from build123d import *

# Parameters (mm, degrees)
F1_DEPTH = 50.038
F3_W     = 44.874294
F3_H     = 28.605775
F4_DEPTH = 25.4


with BuildPart() as f1:
    # F0 (on Right) → F1 (new body)
    with BuildSketch(Plane.YZ):
        Polygon((-80.399789, 0), (-5.07506, 0), (-17.896298, 47.656219), (-80.399789, 50.697614), align=None)
    extrude(amount=F1_DEPTH)

    # F3 (on face) → F4 (cut)
    with BuildSketch(Plane.YZ.offset(50.038)):
        with Locations((-44.732259, 23.702547)):
            Rectangle(F3_W, F3_H)
    extrude(amount=-F4_DEPTH, mode=Mode.SUBTRACT)


solid = f1.part
Could you check a few things on this model? Use its own coordinates, in mm. A direction names the side the tool comes from. Round coordinates to 2 decimals unless told otherwise and drop trailing zeros. Loops run counter-clockwise (first coordinate to the right, second up) from the corner with the lowest first, then second, coordinate; pieces in that order, holes last. Notation, with made-up numbers: (17, 73) -> (37, 73) arc R19 cw to (37, 99) -> close; hole circle Ø6 at (62.25, 3). An arc over 180 degrees is marked (long way). Use CSV: the item, a comma, the result in double quotes.
(1) If I drill on probe 1 along X at (y, z) = (-28, 31.5); probe 2 along Z at (x, y) = (33, -30); probe 3 along Y at (x, z) = (28.5, 13.5), over which ranges is the centre line in solid material (lowest first)? Write a range as [from, to].
Return value:
probe 1,"x = [0, 24.64]"
probe 2,"z = [0, 9.4], [38.01, 48.25]"
probe 3,"y = [-80.4, -67.17], [-22.3, -8.71]"
(2) For faces 1 (the flat face through (0, -43, 26)), 2 (the flat face through (38, -67.169, 24)), which set-ups out of +Z, -Z, +X, -X, +Y, -Y let a thin tool reach every point of the face, with its end or its side?
Return value:
face 1,"+Z, -Z, -X, +Y, -Y"
face 2,"+X"
(3) Will these pins go through, and if not, where does the flat tip stop? pin 1 Ø7.5 at (x, z) = (39, 22) entering from +Y; pin 2 Ø1.5 at (x, y) = (31, -50) entering from -Z; pin 3 Ø4 at (x, z) = (42, 24) entering from +Y; pin 4 Ø10 at (x, z) = (42, 23) entering from +Y.
Return value:
pin 1,"stops at y = -9.98"
pin 2,"stops at z = 0"
pin 3,"stops at y = -10.99"
pin 4,"stops at y = -9.92"
(4) Suppose I cut it at A-A on x = 33. Write out the boundary of the cut face in (y, z), plus the area to 3 significant figures.
Return value:
outline,"(-80.4, 0) -> (-5.08, 0) -> (-17.9, 47.66) -> (-80.4, 50.7) -> close; hole (-67.17, 9.4) -> (-22.3, 9.4) -> (-22.3, 38.01) -> (-67.17, 38.01) -> close"
area,"2,100 mm²"
(5) Suppose I cut it at D-D on x = 20.5. Write out the boundary of the cut face in (y, z).
Return value:
outline,"(-80.4, 0) -> (-5.08, 0) -> (-17.9, 47.66) -> (-80.4, 50.7) -> close"
(6) If we mould it in two halves opening along Z, with no side actions, what happens to faces 3 (the flat face through (24.669, -11.396, 23.495)), 4 (the flat face through (50.038, -52, 9)), 5 (the flat face through (24.638, -45, 24)), 6 (the flat face through (25, -43, 0))? For each: +Z half, -Z half, draft (parallel to the pull), parting line (faces both ways), or undercut.
Return value:
face 3,"+Z half"
face 4,"draft"
face 5,"undercut"
face 6,"-Z half"
(7) Suppose I cut it at C-C on z = 31. Write out the boundary of the cut face in (x, y), plus the area to 3 significant figures.
Return value:
outline,"(0, -80.4) -> (50.04, -80.4) -> (50.04, -67.17) -> (24.64, -67.17) -> (24.64, -22.3) -> (50.04, -22.3) -> (50.04, -13.42) -> (0, -13.42) -> close"
area,"2,210 mm²"
(8) Suppose I cut it at B-B on y = -36. Write out the boundary of the cut face in (x, z).
Return value:
outline,"(0, 0) -> (50.04, 0) -> (50.04, 9.4) -> (24.64, 9.4) -> (24.64, 38.01) -> (50.04, 38.01) -> (50.04, 48.54) -> (0, 48.54) -> close"
